from build123d import *

# Parameters (mm, degrees)
BOSS_EXTRU_1_DEPTH       = 132
ESQUISSE3_W              = 4.94012132
ESQUISSE3_H              = 40
ENL_V_MAT_EXTRU_2_DEPTH  = 9
ESQUISSE4_R              = 1.3
ENL_V_MAT_EXTRU_3_DEPTH  = 18
ESQUISSE5_W              = 6
ESQUISSE5_H              = 24
ENL_V_MAT_EXTRU_4_DEPTH  = 8
BOSS_EXTRU_2_REACH       = 38.8
ESQUISSE7_W              = 2
ESQUISSE7_H              = 18
ENL_V_MAT_EXTRU_5_DEPTH  = 15
ENL_V_MAT_EXTRU_6_DEPTH  = 15
ESQUISSE10_W             = 5.625
ESQUISSE10_H             = 32
BOSS_EXTRU_3_DEPTH       = 17
ESQUISSE14_W             = 11.349962924
ESQUISSE14_H             = 7.588006138
BOSS_EXTRU_5_DEPTH       = 6
ESQUISSE16_W             = 13.258712606
ESQUISSE16_H             = 4.272246905
ENL_V_MAT_EXTRU_7_DEPTH  = 11
ESQUISSE17_W             = 15.613345165
ESQUISSE17_H             = 5.100882875
BOSS_EXTRU_6_DEPTH       = 11
BOSS_EXTRU_6_DEPTH_BACK  = 11
ESQUISSE11_R             = 1.85
ESQUISSE11_R_2           = 1.3
ESQUISSE11_R_3           = 2.916438904
ENL_V_MAT_EXTRU_8_DEPTH  = 8
ESQUISSE18_W             = 9.677736186
ESQUISSE18_H             = 8.253244783
ENL_V_MAT_EXTRU_9_DEPTH  = 10
CONG_2_R                 = 5
ESQUISSE20_W             = 27.3
ESQUISSE20_H             = 40.032665724
ENL_V_MAT_EXTRU_11_DEPTH = 22
ESQUISSE22_R             = 2.780350547
ENL_V_MAT_EXTRU_12_DEPTH = 33
ENL_V_MAT_EXTRU_13_DEPTH = 23
ESQUISSE24_W             = 101.568694303
ESQUISSE24_H             = 64.896510992
ENL_V_MAT_EXTRU_14_DEPTH = 80


with BuildPart() as part:
    # Esquisse1 → Boss.-Extru.1 (new body)
    with BuildSketch(Plane.XY):
        with BuildLine():
            Line((-12.4, 0), (-18.4, 0))
            Line((-18.4, 0), (-18.4, 18))
            Line((-18.4, 18), (18.4, 18))
            Line((18.4, 18), (18.4, 0))
            Line((18.4, 0), (12.4, 0))
            ThreePointArc((12.4, 0), (0, 12.4), (-12.4, 0))
        make_face()
    extrude(amount=BOSS_EXTRU_1_DEPTH)

    # Esquisse3 → Enlèv. mat.-Extru.2 (cut)
    with BuildSketch(Plane.XZ.offset(-18)):
        with Locations((0, 66)):
            Rectangle(ESQUISSE3_W, ESQUISSE3_H)
    extrude(amount=ENL_V_MAT_EXTRU_2_DEPTH, mode=Mode.SUBTRACT)

    # Esquisse4 → Enlèv. mat.-Extru.3 (cut)
    with BuildSketch(Plane(origin=(0, 18, 0), x_dir=(1, 0, 0), z_dir=(0, 1, 0))):
        with Locations((15.4, -6)):
            Circle(ESQUISSE4_R)
        with Locations((15.4, -18)):
            Circle(ESQUISSE4_R)
        with Locations((-15.4, -6)):
            Circle(ESQUISSE4_R)
        with Locations((-15.4, -18)):
            Circle(ESQUISSE4_R)
        with Locations((15.4, -30)):
            Circle(ESQUISSE4_R)
        with Locations((-15.4, -30)):
            Circle(ESQUISSE4_R)
        with Locations((15.4, -42)):
            Circle(ESQUISSE4_R)
        with Locations((-15.4, -42)):
            Circle(ESQUISSE4_R)
        with Locations((-15.4, -126)):
            Circle(ESQUISSE4_R)
        with Locations((-15.4, -114)):
            Circle(ESQUISSE4_R)
        with Locations((-15.4, -102)):
            Circle(ESQUISSE4_R)
        with Locations((-15.4, -90)):
            Circle(ESQUISSE4_R)
        with Locations((-15.4, -78)):
            Circle(ESQUISSE4_R)
        with Locations((15.4, -78)):
            Circle(ESQUISSE4_R)
        with Locations((15.4, -90)):
            Circle(ESQUISSE4_R)
        with Locations((15.4, -102)):
            Circle(ESQUISSE4_R)
        with Locations((15.4, -114)):
            Circle(ESQUISSE4_R)
        with Locations((15.4, -126)):
            Circle(ESQUISSE4_R)
    extrude(amount=-ENL_V_MAT_EXTRU_3_DEPTH, mode=Mode.SUBTRACT)

    # Esquisse5 → Enlèv. mat.-Extru.4 (cut)
    with BuildSketch(Plane(origin=(0, 18, 0), x_dir=(1, 0, 0), z_dir=(0, 1, 0))):
        with Locations((15.4, -12)):
            Rectangle(ESQUISSE5_W, ESQUISSE5_H)
        with Locations((-15.4, -120)):
            Rectangle(ESQUISSE5_W, ESQUISSE5_H)
        with Locations((-15.4, -12)):
            Rectangle(ESQUISSE5_W, ESQUISSE5_H)
        with Locations((15.4, -120)):
            Rectangle(ESQUISSE5_W, ESQUISSE5_H)
    extrude(amount=-ENL_V_MAT_EXTRU_4_DEPTH, mode=Mode.SUBTRACT)

    # Esquisse7 → Boss.-Extru.2 (add, up to next)
    with BuildSketch(Plane.ZY.offset(18.4), mode=Mode.PRIVATE) as boss_extru_2_sk1:
        with Locations((66, 9)):
            Rectangle(ESQUISSE7_W, ESQUISSE7_H)
    boss_extru_2_tool1 = extrude(boss_extru_2_sk1.sketch, amount=-BOSS_EXTRU_2_REACH, mode=Mode.PRIVATE) - part.part
    add(boss_extru_2_tool1.solids().sort_by_distance((-18.4, 9, 66))[0])

    # Esquisse8 → Enlèv. mat.-Extru.5 (cut)
    with BuildSketch(Plane(origin=(0, 0, 65), x_dir=(-1, 0, 0), z_dir=(0, 0, -1))):
        with BuildLine():
            Line((12.775, 0), (-12.775, 0))
            ThreePointArc((-12.775, 0), (0, 12.775), (12.775, 0))
        make_face()
    extrude(amount=ENL_V_MAT_EXTRU_5_DEPTH, mode=Mode.SUBTRACT)

    # Esquisse9 → Enlèv. mat.-Extru.6 (cut)
    with BuildSketch(Plane.XY.offset(67)):
        with BuildLine():
            Line((12.775, 0), (-12.775, 0))
            ThreePointArc((-12.775, 0), (0, 12.775), (12.775, 0))
        make_face()
    extrude(amount=ENL_V_MAT_EXTRU_6_DEPTH, mode=Mode.SUBTRACT)

    # Esquisse10 → Boss.-Extru.3 (add)
    with BuildSketch(Plane.XZ):
        with Locations((15.5875, 66)):
            Rectangle(ESQUISSE10_W, ESQUISSE10_H)
        with Locations((-15.5875, 66)):
            Rectangle(ESQUISSE10_W, ESQUISSE10_H)
    extrude(amount=BOSS_EXTRU_3_DEPTH)

    # Esquisse14 → Boss.-Extru.5 (add)
    with BuildSketch(Plane(origin=(18.4, 0, 0), x_dir=(0, 0, -1), z_dir=(1, 0, 0))):
        with Locations((-50.7944077, 14.205996931)):
            Rectangle(ESQUISSE14_W, ESQUISSE14_H)
    extrude(amount=BOSS_EXTRU_5_DEPTH)

    # Esquisse16 → Enlèv. mat.-Extru.7 (cut)
    with BuildSketch(Plane(origin=(24.4, 0, 0), x_dir=(0, 0, -1), z_dir=(1, 0, 0))):
        with Locations((-50.566594151, 10.91391733)):
            Rectangle(ESQUISSE16_W, ESQUISSE16_H)
    extrude(amount=-ENL_V_MAT_EXTRU_7_DEPTH, mode=Mode.SUBTRACT)

    # Esquisse17 → Boss.-Extru.6 (add, two sides)
    with BuildSketch(Plane(origin=(18.4, 0, 0), x_dir=(0, 0, -1), z_dir=(1, 0, 0))) as boss_extru_6_sk:
        with Locations((-21.308135783, 15.449558563)):
            Rectangle(ESQUISSE17_W, ESQUISSE17_H)
    extrude(amount=BOSS_EXTRU_6_DEPTH)
    extrude(boss_extru_6_sk.sketch, amount=-BOSS_EXTRU_6_DEPTH_BACK)

    # Esquisse11 → Enlèv. mat.-Extru.8 (cut)
    with BuildSketch(Plane(origin=(0, 18, 0), x_dir=(1, 0, 0), z_dir=(0, 1, 0))):
        with Locations((24.22, -102)):
            Circle(ESQUISSE11_R)
        with Locations((19.13, -51)):
            Circle(ESQUISSE11_R)
        with Locations((24.22, -20.6)):
            Circle(ESQUISSE11_R)
        with Locations((-8.37, -51)):
            Circle(ESQUISSE11_R)
        with Locations((15.4, -6)):
            Circle(ESQUISSE11_R_2)
        with Locations((15.4, -18)):
            Circle(ESQUISSE11_R_3)
        with Locations((-23.98, -101)):
            Circle(ESQUISSE11_R)
        with Locations((-23.98, -28)):
            Circle(ESQUISSE11_R)
    extrude(amount=-ENL_V_MAT_EXTRU_8_DEPTH, mode=Mode.SUBTRACT)

    # Esquisse18 → Enlèv. mat.-Extru.9 (cut)
    with BuildSketch(Plane(origin=(-2.47006066, 0, 0), x_dir=(0, 0, -1), z_dir=(1, 0, 0))):
        with Locations((-50.900131157, 9.01339788)):
            Rectangle(ESQUISSE18_W, ESQUISSE18_H)
    extrude(amount=-ENL_V_MAT_EXTRU_9_DEPTH, mode=Mode.SUBTRACT)

    # Congé2
    cong_2_edges = [part.edges().sort_by_distance(p)[0] for p in [
        (0, 18, 0),
        (0, 18, 132),
    ]]
    fillet(cong_2_edges, radius=CONG_2_R)

    # Esquisse20 → Enlèv. mat.-Extru.11 (cut)
    with BuildSketch(Plane.XZ):
        with Locations((0, 66)):
            Rectangle(ESQUISSE20_W, ESQUISSE20_H)
    extrude(amount=ENL_V_MAT_EXTRU_11_DEPTH, mode=Mode.SUBTRACT)

    # Esquisse22 → Enlèv. mat.-Extru.12 (cut)
    with BuildSketch(Plane.XZ.offset(-13.050040782)):
        with Locations((19.13, 51)):
            Circle(ESQUISSE22_R)
    extrude(amount=ENL_V_MAT_EXTRU_12_DEPTH, mode=Mode.SUBTRACT)

    # Esquisse23 → Enlèv. mat.-Extru.13 (cut)
    with BuildSketch(Plane.XZ.offset(-13.140020271)):
        Polygon((-10.962659815, 54.736061467), (-30.574521602, 60.209177611), (-30.574521602, 54.651975737), (-10.962659815, 50.396101529), align=None)
    extrude(amount=ENL_V_MAT_EXTRU_13_DEPTH, mode=Mode.SUBTRACT)

    # Esquisse24 → Enlèv. mat.-Extru.14 (cut)
    with BuildSketch(Plane(origin=(0, 0, 65), x_dir=(-1, 0, 0), z_dir=(0, 0, -1))):
        with Locations((-4.820186709, 5.897951476)):
            Rectangle(ESQUISSE24_W, ESQUISSE24_H)
    extrude(amount=ENL_V_MAT_EXTRU_14_DEPTH, mode=Mode.SUBTRACT)


solid = part.part
Build history of the part. All positions in model axes, mm. A direction names the side the tool comes from. Give positions to 0.01 mm unless a question says otherwise; leave off trailing zeros. Loops run counter-clockwise (first coordinate to the right, second up) from the corner with the lowest first, then second, coordinate; pieces in that order, holes last. Notation, with made-up numbers: (66, 58.25) - (80, 58.25) arc R22 ccw to (80, 90.25) - close; hole circle Ø9 at (80.25, -30). An arc over 180 degrees is marked (long way). Write item = value, one per line. Start each with the question number.
1) Probe probe 1 along Z at (x, y) = (-15.4, 12.25); probe 2 along X at (y, z) = (-1, 80); probe 3 along Z at (x, y) = (15, 6). List the from-to ranges inside material, lowest first. Write a range as from..to.
2) Band-saw the part on D-D on y = -9. Give the cut face in (x, z).
3) Drop flat-ended pins along their axis: pin 1 Ø4 at (x, z) = (-6.5, 118) entering from -Y; pin 2 Ø5.5 at (x, y) = (-3, 5) entering from +Z; pin 3 Ø4 at (x, z) = (-15.4, 90) entering from -Y. Give the stop position or say it passes through.
4) Band-saw the part on A-A on x = -15.4. Give the cut face in (y, z).
5) Band-saw the part on B-B on z = 102. Give the cut face in (x, y).
6) Tool access for faces 1 (the cylindrical face through (-9.946, 8.018, 74.395)), 2 (the flat face through (-15, 0, 78)), 3 (the flat face through (-13.65, -8, 73)), 4 (the flat face through (2.47, 15, 76)): list every direction of +Z, -Z, +X, -X, +Y, -Y with a clear straight run to the whole face (end or side of a thin tool).
7) Band-saw the part on C-C on z = 78. Give the cut face in (x, y) (3 decimals), plus the area to 3 significant figures.
8) Pull direction Z, two halves, no side cores. Call faces 5 (the cylindrical face through (-15.57, 5.07, 124.71)), 6 (the flat face through (4, 12, 132)), 7 (the flat face through (-14, 0, 98)): +Z half, -Z half, draft (parallel to the pull), parting line (faces both ways), or undercut.
Final values:
q1.probe_1 = 65..76.7, 79.3..88.7, 91.3..100.7, 103.3..108
q1.probe_2 = -18.4..-13.65, 13.65..18.4
q1.probe_3 = 65..76.76, 79.24..88.76, 91.24..100.76, 103.24..112.76, 115.24..124.76, 127.24..132
q2.outline = (-18.4, 65) - (-13.65, 65) - (-13.65, 82) - (-18.4, 82) - close; (13.65, 65) - (18.4, 65) - (18.4, 82) - (13.65, 82) - close
q3.pin_1 = 9.03
q3.pin_2 = 67
q3.pin_3 = 0
q4.outline = (-17, 65) - (18, 65) - (18, 76.7) - (0, 76.7) - (0, 79.3) - (18, 79.3) - (18, 88.7) - (0, 88.7) - (0, 82) - (-17, 82) - close; (0, 91.3) - (18, 91.3) - (18, 100.7) - (0, 100.7) - close; (0, 103.3) - (18, 103.3) - (18, 108) - (10, 108) - (10, 112.7) - (0, 112.7) - close; (0, 115.3) - (10, 115.3) - (10, 124.7) - (0, 124.7) - close; (0, 127.3) - (10, 127.3) - (10, 132) - (0, 132) - close
q5.outline = (-18.4, 0) - (-16.7, 0) - (-16.7, 18) - (-18.4, 18) - close; (-14.1, 0) - (-12.4, 0) arc R12.4 cw to (12.4, 0) - (14.1, 0) - (14.1, 18) - (-14.1, 18) - close; (16.7, 0) - (18.4, 0) - (18.4, 18) - (16.7, 18) - close
q6.face_1 = -Y
q6.face_2 = +Y
q6.face_3 = +Z, -Z, -Y
q6.face_4 = +Y, -Y
q7.outline = (-18.4, -17) - (-13.65, -17) - (-13.65, 0) - (-12.775, 0) arc R12.775 cw to (-2.47, 12.534) - (-2.47, 18) - (-14.1, 18) - (-14.1, 0) - (-16.7, 0) - (-16.7, 18) - (-18.4, 18) - close; (2.47, 12.534) arc R12.775 cw to (12.775, 0) - (13.65, 0) - (13.65, -17) - (18.4, -17) - (18.4, 18) - (16.7, 18) - (16.7, 0) - (14.1, 0) - (14.1, 18) - (2.47, 18) - close
q7.area = 448 mm²
q8.face_5 = undercut
q8.face_6 = +Z half
q8.face_7 = draft
